Model file for the job. Use its own axes, mm. Face numbers are marked on the shaded views. Round coordinates to 2 decimals unless told otherwise and drop trailing zeros. One line per item, written item: value.
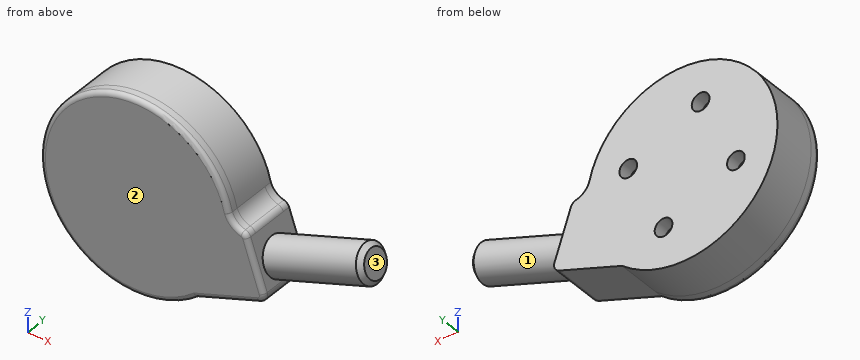
from build123d import *

# Parameters (mm, degrees)
STOCK_REFERENCE_START            = -175.975505736
STOCK_REFERENCE_SEAT_1_OUTLINE_R = 32.264078684
STOCK_REFERENCE_SEAT_1_DEPTH     = 15.311729992
STOCK_REFERENCE_SEAT_1_2_DEPTH   = 12.7
BOSS_EXTRUDE3_START              = 3.738270008
BOSS_EXTRUDE3_DEPTH              = 3.738270008
BOSS_EXTRUDE1_DEPTH              = 2.611729992
SKETCH2_R                        = 6.35
BOSS_EXTRUDE2_DEPTH              = 34.925
CHAMFER1_SIZE                    = 1.5875
FILLET1_R                        = 6.35
FILLET2_R                        = 2.54
FILLET3_R                        = 1.5875
HOLE1_AT_2_COUNT                 = 2
HOLE1_AT_2_PITCH                 = 27.213140303
HOLE1_AT_3_COUNT                 = 2
HOLE1_AT_3_PITCH                 = 38.485192091
HOLE1_AT_4_COUNT                 = 2
HOLE1_AT_4_PITCH                 = 27.213140303
F_8_CLEARANCE_HOLE1_D            = 4.9149
F_8_CLEARANCE_HOLE1_DEPTH        = 12.7
F_8_CLEARANCE_HOLE1_TIP          = 1.476584928


# Read off the part's stored shape, not the designer's step: Stock-Reference Seat-1
with BuildPart() as part:
    # Stock-Reference Seat-1 outline → Stock-Reference Seat-1 (new body)
    with BuildSketch(Plane(origin=(0, 0, 0), x_dir=(1, 0, 0), z_dir=(0, 1, 0)).offset(STOCK_REFERENCE_START)):
        with Locations((-264.046286299, 242.023928087)):
            Circle(STOCK_REFERENCE_SEAT_1_OUTLINE_R)
    extrude(amount=STOCK_REFERENCE_SEAT_1_DEPTH)

    # Stock-Reference Seat-1 2 outline → Stock-Reference Seat-1 2 (add)
    with BuildSketch(Plane(origin=(0, 0, 0), x_dir=(1, 0, 0), z_dir=(0, 1, 0)).offset(STOCK_REFERENCE_START)):
        with BuildLine():
            ThreePointArc((-243.756619182, 267.109784294), (-233.536149053, 252.516892329), (-232.618762484, 234.724508918))
            Line((-232.618762484, 234.724508918), (-230.711355396, 240.263016846))
            Line((-230.711355396, 240.263016846), (-226.943146121, 238.965283021))
            Line((-226.943146121, 238.965283021), (-220.060881103, 258.949207593))
            Line((-220.060881103, 258.949207593), (-243.756619182, 267.109784294))
        make_face()
    extrude(amount=STOCK_REFERENCE_SEAT_1_2_DEPTH)

    # Sketch7 → Boss-Extrude3 (add)
    with BuildSketch(Plane.XZ.offset(175.975505736).offset(BOSS_EXTRUDE3_START)):
        with BuildLine():
            Line((-243.756619182, -267.109784294), (-220.060881103, -258.949207593))
            Line((-220.060881103, -258.949207593), (-226.943146121, -238.965283021))
            Line((-226.943146121, -238.965283021), (-230.711355396, -240.263016846))
            Line((-230.711355396, -240.263016846), (-232.618762484, -234.724508918))
            ThreePointArc((-232.618762484, -234.724508918), (-294.556423545, -231.530963846), (-243.756619182, -267.109784294))
        make_face()
    extrude(amount=-BOSS_EXTRUDE3_DEPTH)

    # Sketch1 → Boss-Extrude1 (add)
    with BuildSketch(Plane(origin=(0, -163.275505736, 0), x_dir=(1, 0, 0), z_dir=(0, 1, 0))):
        with BuildLine():
            Line((-232.618762484, 234.724508918), (-230.711355396, 240.263016846))
            Line((-230.711355396, 240.263016846), (-226.943146121, 238.965283021))
            Line((-226.943146121, 238.965283021), (-220.060881103, 258.949207593))
            Line((-220.060881103, 258.949207593), (-243.756619182, 267.109784294))
            ThreePointArc((-243.756619182, 267.109784294), (-233.536149053, 252.516892329), (-232.618762484, 234.724508918))
        make_face()
    extrude(amount=BOSS_EXTRUDE1_DEPTH)

    # Sketch2 → Boss-Extrude2 (add)
    with BuildSketch(Plane(origin=(-276.451963722, 0, -95.207308867), x_dir=(0.325620940566074, 0, -0.9455003982362278), z_dir=(0.9455003982362278, 0, 0.32562094056607405))):
        with Locations((163.652309847, -170.188775744)):
            Circle(SKETCH2_R)
    extrude(amount=BOSS_EXTRUDE2_DEPTH)

    # Chamfer1
    chamfer1_edges = [part.edges().sort_by_distance(p)[0] for p in [
        (-192.209436228, -170.188775744, -232.564394121),
    ]]
    chamfer(chamfer1_edges, length=CHAMFER1_SIZE)

    # Fillet1
    # the kernel refuses this fillet: 6.35 mm, written as the material it adds along each edge
    with BuildSketch(Plane(origin=(-230.711355396, -175.975505736, -240.263016846), x_dir=(0.9455003982389363, 0, 0.3256209405582093), z_dir=(0, 1, 0))) as fillet1_piece_1:
        with BuildLine():
            CenterArc((6.349999999, -5.893320524), FILLET1_R, 111.862223466, 68.137776529)
            Line((-1e-09, -5.893320524), (-0.127000001, -5.893320524))
            Line((-0.127000001, -5.893320524), (-0.127, 0))
            Line((-0.127, 0), (0, 0.127))
            ThreePointArc((0, 0.127), (1.992706339, 0.127), (3.938120932, 0.11786641))
            Line((3.938120932, 0.11786641), (3.985412679, 0))
        make_face()
    extrude(amount=12.7)
    with BuildSketch(Plane(origin=(-230.711355396, -179.713775744, -240.263016846), x_dir=(0.9455003982362268, 0, 0.3256209405660767), z_dir=(0, 1, 0))) as fillet1_piece_2:
        with BuildLine():
            CenterArc((6.35, -5.893320524), FILLET1_R, 111.862223465, 68.137776535)
            Line((0, -5.893320524), (-0.127, -5.893320524))
            Line((-0.127, -5.893320524), (-0.127, 0))
            Line((-0.127, 0), (0, 0.127))
            ThreePointArc((0, 0.127), (1.99270634, 0.127), (3.938120933, 0.11786641))
            Line((3.938120933, 0.11786641), (3.98541268, 0))
        make_face()
    extrude(amount=3.738270008)
    with BuildSketch(Plane(origin=(-230.711355396, -163.275505736, -240.263016846), x_dir=(0.9455003982362268, 0, 0.3256209405660767), z_dir=(0, 1, 0))) as fillet1_piece_3:
        with BuildLine():
            CenterArc((6.35, -5.893320524), FILLET1_R, 111.862223465, 68.137776535)
            Line((0, -5.893320524), (-0.127, -5.893320524))
            Line((-0.127, -5.893320524), (-0.127, 0))
            Line((-0.127, 0), (0, 0.127))
            ThreePointArc((0, 0.127), (1.99270634, 0.127), (3.938120933, 0.11786641))
            Line((3.938120933, 0.11786641), (3.98541268, 0))
        make_face()
    extrude(amount=2.611729992)

    # Fillet2
    fillet2_edges = [part.edges().sort_by_distance(p)[0] for p in [
        (-226.943146121, -169.625505736, -238.965283021),
        (-220.060881103, -169.625505736, -258.949207593),
    ]]
    fillet(fillet2_edges, radius=FILLET2_R)

    # Fillet3
    fillet3_edges = [part.edges().sort_by_distance(p)[0] for p in [
        (-233.109535648, -179.713775744, -263.443034538),
        (-294.55657248, -179.713775744, -231.531396911),
        (-223.667862866, -179.713775744, -248.475671438),
        (-230.923127248, -179.713775744, -237.298737872),
        (-227.125556964, -179.713775744, -239.36526013),
        (-221.006530266, -179.713775744, -258.488049029),
    ]]
    fillet(fillet3_edges, radius=FILLET3_R)

    # Sketch4 → Hole1 (revolve, cut)
    with BuildSketch(Plane(origin=(-245.852404075, -160.663775744, -235.758135864), x_dir=(0, 0, 1), z_dir=(1, 0, 0))):
        Polygon((0, 0), (0, 4.699), (2.8702, 4.699), (2.9972, 0), align=None)
    hole1 = revolve(axis=Axis((-245.852404075, -270.663775744, -235.758135864), (0, 1, 0)), mode=Mode.SUBTRACT)

    # Hole1 at 2: Hole1 ×2
    with Locations(*[Vector(-0.8988185183780313, 0, 0.43832096803680365) * (i * HOLE1_AT_2_PITCH) for i in range(1, HOLE1_AT_2_COUNT)]):
        add(hole1, mode=Mode.SUBTRACT)

    # Hole1 at 3: Hole1 ×2
    with Locations(*[Vector(-0.945500398236235, 0, -0.3256209405660531) * (i * HOLE1_AT_3_PITCH) for i in range(1, HOLE1_AT_3_COUNT)]):
        add(hole1, mode=Mode.SUBTRACT)

    # Hole1 at 4: Hole1 ×2
    with Locations(*[Vector(-0.4383209680367791, 0, -0.8988185183780433) * (i * HOLE1_AT_4_PITCH) for i in range(1, HOLE1_AT_4_COUNT)]):
        add(hole1, mode=Mode.SUBTRACT)

    # #8 Clearance Hole1
    with Locations(Plane(origin=(0, -160.663775744, 0), x_dir=(1, 0, 0), z_dir=(0, 1, 0))):
        with Locations((-245.852404075, 235.758135864), (-270.312078522, 223.830045863), (-282.240168523, 248.289720311), (-257.780494076, 260.217810311)):
            Hole(F_8_CLEARANCE_HOLE1_D / 2, depth=F_8_CLEARANCE_HOLE1_DEPTH)
            with Locations((0, 0, -(F_8_CLEARANCE_HOLE1_DEPTH + F_8_CLEARANCE_HOLE1_TIP / 2))):  # 118° drill point
                Cone(0, F_8_CLEARANCE_HOLE1_D / 2, F_8_CLEARANCE_HOLE1_TIP, mode=Mode.SUBTRACT)


solid = part.part
1. Wall check: probe 1 along Z at (x, y) = (-254, -176); probe 2 along Y at (x, z) = (-248, -234.5); probe 3 along X at (y, z) = (-166.5, -224). Give the ranges that are in metal, low to high. Write a range as [from, to].
Report:
probe 1: [-272.68, -211.36]
probe 2: [-179.71, -165.36]
probe 3: [-290.81, -272.76], [-267.86, -237.29]
2. Drop flat-ended pins along their axis: pin 1 (5 mm diameter, centred on x = -211, z = -248.5, fed in from -Y); pin 2 (3 mm diameter, centred on y = -170.5, z = -221, fed in from -X); pin 3 (4 mm diameter, centred on x = -242, y = -168.5, fed in from -Z). Give the stop position or say it passes through.
Report:
pin 1: y = -176.54
pin 2: x = -289.73
pin 3: z = -267.3
3. Mould opens along X. For the marked faces 1, 2 and 3 say: released by +X, released by -X, zero draft, split by the parting line, or undercut.
Report:
face 1: undercut
face 2: zero draft
face 3: released by +X
4. Band-saw the part on A-A on y = -167. State how many separate pieces and enclosed holes the cut face has, plus the area to 3 significant figures.
Report:
separate pieces: 1
enclosed holes: 4
area: 3,830 mm²
